from build123d import *

# Parameters (mm, degrees)
SKETCH1_W           = 70
SKETCH1_H           = 120
BOSS_EXTRUDE1_DEPTH = 1.1
SKETCH2_W           = 70
SKETCH2_H           = 120
SKETCH2_W_2         = 67.6
SKETCH2_H_2         = 117.6
BOSS_EXTRUDE2_DEPTH = 7
SKETCH3_W           = 1.2
SKETCH3_H           = 3
BOSS_EXTRUDE3_DEPTH = 4.5
SKETCH5_W           = 0.8
SKETCH5_H           = 1
BOSS_EXTRUDE4_DEPTH = 3
SKETCH6_W           = 0.8
SKETCH6_H           = 1
BOSS_EXTRUDE5_DEPTH = 3
SKETCH7_W           = 7
SKETCH7_H           = 1.2
CUT_EXTRUDE1_DEPTH  = 3
SKETCH8_W           = 1
SKETCH8_H           = 7
BOSS_EXTRUDE6_DEPTH = 2
FILLET1_SIZE        = 1.5
FILLET2_SIZE        = 1.2
FILLET3_R           = 0.8
FILLET4_R           = 3


# Some blends are built 0.0001 mm under size
with BuildPart() as part:
    # Sketch1 → Boss-Extrude1 (new body)
    with BuildSketch(Plane(origin=(0, 0, 0), x_dir=(1, 0, 0), z_dir=(0, 1, 0))):
        with Locations((35, -60)):
            Rectangle(SKETCH1_W, SKETCH1_H)
    extrude(amount=BOSS_EXTRUDE1_DEPTH)

    # Sketch2 → Boss-Extrude2 (add)
    with BuildSketch(Plane(origin=(0, 1.1, 0), x_dir=(1, 0, 0), z_dir=(0, 1, 0))):
        with Locations((35, -60)):
            Rectangle(SKETCH2_W, SKETCH2_H)
        with Locations((35, -60)):
            Rectangle(SKETCH2_W_2, SKETCH2_H_2, mode=Mode.SUBTRACT)
    extrude(amount=BOSS_EXTRUDE2_DEPTH)

    # Sketch3 → Boss-Extrude3 (add)
    with BuildSketch(Plane(origin=(0, 1.1, 0), x_dir=(1, 0, 0), z_dir=(0, 1, 0))):
        with Locations((57.5, -13.5)):
            Rectangle(SKETCH3_W, SKETCH3_H)
        with Locations((12.5, -13.5)):
            Rectangle(SKETCH3_W, SKETCH3_H)
        with Locations((57.5, -106.5)):
            Rectangle(SKETCH3_W, SKETCH3_H)
        with Locations((12.5, -106.5)):
            Rectangle(SKETCH3_W, SKETCH3_H)
    extrude(amount=BOSS_EXTRUDE3_DEPTH)

    # Sketch5 → Boss-Extrude4 (add)
    with BuildSketch(Plane(origin=(0, 0, 12), x_dir=(-1, 0, 0), z_dir=(0, 0, -1))):
        with Locations((-56.5, 5.1)):
            Rectangle(SKETCH5_W, SKETCH5_H)
        with Locations((-13.5, 5.1)):
            Rectangle(SKETCH5_W, SKETCH5_H)
    extrude(amount=-BOSS_EXTRUDE4_DEPTH)

    # Sketch6 → Boss-Extrude5 (add)
    with BuildSketch(Plane(origin=(0, 0, 105), x_dir=(-1, 0, 0), z_dir=(0, 0, -1))):
        with Locations((-56.5, 5.1)):
            Rectangle(SKETCH6_W, SKETCH6_H)
        with Locations((-13.5, 5.1)):
            Rectangle(SKETCH6_W, SKETCH6_H)
    extrude(amount=-BOSS_EXTRUDE5_DEPTH)

    # Sketch7 → Cut-Extrude1 (cut)
    with BuildSketch(Plane(origin=(0, 8.1, 0), x_dir=(1, 0, 0), z_dir=(0, 1, 0))):
        with Locations((52.5, -0.6)):
            Rectangle(SKETCH7_W, SKETCH7_H)
        with Locations((17.5, -0.6)):
            Rectangle(SKETCH7_W, SKETCH7_H)
    extrude(amount=-CUT_EXTRUDE1_DEPTH, mode=Mode.SUBTRACT)

    # Sketch8 → Boss-Extrude6 (add)
    with BuildSketch(Plane(origin=(0, 0, 118.8), x_dir=(-1, 0, 0), z_dir=(0, 0, -1))):
        with Locations((-49.5, 4.6)):
            Rectangle(SKETCH8_W, SKETCH8_H)
        with Locations((-20.5, 4.6)):
            Rectangle(SKETCH8_W, SKETCH8_H)
    extrude(amount=BOSS_EXTRUDE6_DEPTH)

    # Fillet1
    # a fillet whose section is not a circle: 1.5 mm, written as the material it adds along each edge
    with BuildSketch(Plane(origin=(13.1, 1.1, 15), x_dir=(1, 0, 0), z_dir=(0, 0, -1))) as fillet1_piece_1:
        with BuildLine():
            Bezier((FILLET1_SIZE, 0), (0, 0), (0, -FILLET1_SIZE), weights=[1, 0.111111111, 1])
            Line((0, -FILLET1_SIZE), (0, 0))
            Line((0, 0), (FILLET1_SIZE, 0))
        make_face()
    extrude(amount=3)
    with BuildSketch(Plane(origin=(56.9, 1.1, 15), x_dir=(-1, 0, 0), z_dir=(0, 0, -1)), Plane(origin=(56.9, 1.1, 108), x_dir=(-1, 0, 0), z_dir=(0, 0, -1)), Plane(origin=(13.1, 1.1, 105), x_dir=(1, 0, 0), z_dir=(0, 0, 1))) as fillet1_piece_2:
        with BuildLine():
            Bezier((FILLET1_SIZE, 0), (0, 0), (0, FILLET1_SIZE), weights=[1, 0.111111111, 1])
            Line((0, FILLET1_SIZE), (0, 0))
            Line((0, 0), (FILLET1_SIZE, 0))
        make_face()
    extrude(amount=3)

    # Fillet2
    # a fillet whose section is not a circle: 1.2 mm, written as the material it adds along each edge
    with BuildSketch(Plane(origin=(11.9, 1.1, 12), x_dir=(-1, 0, 0), z_dir=(0, 0, 1)), Plane(origin=(58.1, 1.1, 12), x_dir=(0, 1, 0), z_dir=(0, 0, 1))) as fillet2_piece_1:
        with BuildLine():
            Bezier((FILLET2_SIZE, 0), (0, 0), (0, -FILLET2_SIZE), weights=[1, 0.111111111, 1])
            Line((0, -FILLET2_SIZE), (-FILLET2_SIZE * 0.02, -FILLET2_SIZE))
            Line((-FILLET2_SIZE * 0.02, -FILLET2_SIZE), (-FILLET2_SIZE * 0.02, FILLET2_SIZE * 0.02))
            Line((-FILLET2_SIZE * 0.02, FILLET2_SIZE * 0.02), (FILLET2_SIZE, FILLET2_SIZE * 0.02))
            Line((FILLET2_SIZE, FILLET2_SIZE * 0.02), (FILLET2_SIZE, 0))
        make_face()
    extrude(amount=3)
    with BuildSketch(Plane(origin=(58.1, 1.1, 105), x_dir=(1, 0, 0), z_dir=(0, 0, 1)), Plane(origin=(11.9, 1.1, 108), x_dir=(-1, 0, 0), z_dir=(0, 0, -1))) as fillet2_piece_2:
        with BuildLine():
            Bezier((FILLET2_SIZE, 0), (0, 0), (0, FILLET2_SIZE), weights=[1, 0.111111111, 1])
            Line((0, FILLET2_SIZE), (-FILLET2_SIZE * 0.02, FILLET2_SIZE))
            Line((-FILLET2_SIZE * 0.02, FILLET2_SIZE), (-FILLET2_SIZE * 0.02, -FILLET2_SIZE * 0.02))
            Line((-FILLET2_SIZE * 0.02, -FILLET2_SIZE * 0.02), (FILLET2_SIZE, -FILLET2_SIZE * 0.02))
            Line((FILLET2_SIZE, -FILLET2_SIZE * 0.02), (FILLET2_SIZE, 0))
        make_face()
    extrude(amount=3)

    # Fillet3
    fillet3_edges = [part.edges().sort_by_distance(p)[0] for p in [
        (56.9, 4.6, 106.5),
        (56.9, 4.6, 13.5),
        (13.1, 4.6, 13.5),
        (13.1, 4.6, 106.5),
    ]]
    fillet(fillet3_edges, radius=FILLET3_R - 0.0001)  # a hair under: the kernel refuses the full size

    # Fillet4
    fillet4_edges = [part.edges().sort_by_distance(p)[0] for p in [
        (1.2, 1.1, 60),
        (68.8, 1.1, 60),
        (70, 0, 60),
        (0, 0, 60),
    ]]
    fillet(fillet4_edges, radius=FILLET4_R)


solid = part.part
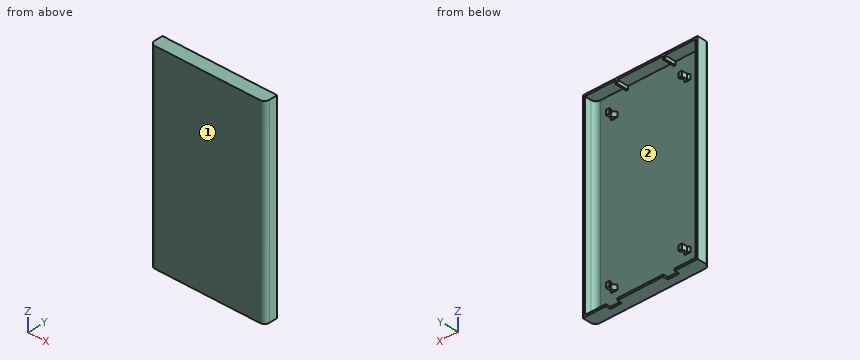
Source: CAD feature listing. Evaluate the final solid. Frame: model axes, mm. Face numbers are marked on the shaded views. Round coordinates to 2 decimals unless told otherwise and drop trailing zeros. Write each loop counter-clockwise with the first axis right and the second up, starting at its lowest first coordinate (ties: lowest second). Pieces come first, ordered by that corner, then holes. Notation, with made-up numbers: (33.25, 49.5) - (57.25, 49.5) arc R14 cw to (57.25, 66.5) - close; hole circle Ø6 at (62.5, 56). An arc over 180 degrees is marked (long way). Use CSV: the item, a comma, the result in double quotes. Start each with the question number.
(1) First-contact query: pin 1 Ø1.1 at (x, y) = (49.5, 6) entering from -Z; pin 2 Ø6 at (x, z) = (30.5, 81.5) entering from +Y; pin 3 Ø0.6 at (x, z) = (57.5, 106.5) entering from +Y. Flat tips, straight axial feed; report the tip coordinate or a pass-through.
(2) Cut plane B-B, the plane z = 32.5. Return loops of the section in (x, y).
(3) Cut plane A-A, the plane x = 63.5. Return loops of the section in (y, z), and give its area (3 significant figures).
(4) Material intervals for probe 1 along Z at (x, y) = (12, 3.25); probe 2 along Z at (x, y) = (34, 5.75); probe 3 along X at (y, z) = (4.5, 18), sorted ascending. Write a range as [from, to].
(5) Mould query, pull axis X, two halves, no side actions, for the marked faces 1 and 2. Classes: pulls with the +X half, pulls with the -X half, needs draft (parallel to the pull), parting line crosses it, or undercut.
Geometry says:
1,pin 1,"z = 0"
1,pin 2,"y = 1.1"
1,pin 3,"y = 5.6"
2,outline,"(0, 3) arc R3 ccw to (3, 0) - (67, 0) arc R3 ccw to (70, 3) - (70, 8.1) - (68.8, 8.1) - (68.8, 4.1) arc R3 cw to (65.8, 1.1) - (4.2, 1.1) arc R3 cw to (1.2, 4.1) - (1.2, 8.1) - (0, 8.1) - close"
3,outline,"(0, 0) - (8.1, 0) - (8.1, 1.2) - (1.1, 1.2) - (1.1, 118.8) - (8.1, 118.8) - (8.1, 120) - (0, 120) - close"
3,area,"149 mm²"
4,probe 1,"[0, 1.2], [12, 15], [105, 108], [118.8, 120]"
4,probe 2,"[0, 1.2], [118.8, 120]"
4,probe 3,"[0, 1.2], [68.8, 70]"
5,face 1,"needs draft"
5,face 2,"undercut"
